Design review of the part built by this model. Coordinates are the model's own, in mm. Face numbers are marked on the shaded views. A direction names the side the tool comes from. Give positions to 0.01 mm unless a question says otherwise; leave off trailing zeros. Write each loop counter-clockwise with the first axis right and the second up, starting at its lowest first coordinate (ties: lowest second). Pieces come first, ordered by that corner, then holes. Notation, with made-up numbers: (42, 20) -> (80, 20) arc R17 ccw to (80, 50) -> close; hole circle Ø5 at (10.5, 36). An arc over 180 degrees is marked (long way). Answer as a JSON object with one key per item and string values.
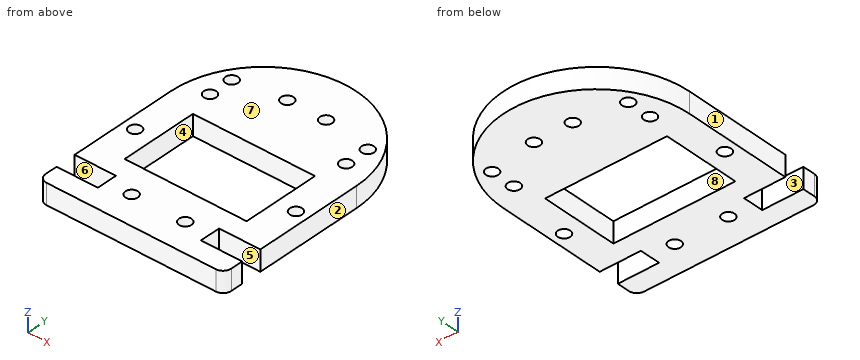
```python
from build123d import *

# Parameters (mm, degrees)
RESSALTO_EXTRUS_O2_DEPTH = 5
ESBO_O9_W                = 29.58
ESBO_O9_H                = 18.85
CORTE_EXTRUS_O1_DEPTH    = 5
ESBO_O10_R               = 1.5
CORTE_EXTRUS_O2_DEPTH    = 5
ESBO_O12_R               = 1.5
CORTE_EXTRUS_O3_DEPTH    = 10
ESBO_O13_R               = 1.5
CORTE_EXTRUS_O4_DEPTH    = 10
ESBO_O14_R               = 1.5
CORTE_EXTRUS_O5_DEPTH    = 76


with BuildPart() as part:
    # Esboço8 → Ressalto-extrusão2 (new body)
    with BuildSketch(Plane.XY):
        with BuildLine():
            Line((-24.266341706, -3.25), (-24.266341706, 13.25))
            ThreePointArc((-24.266341706, 13.25), (-1.766341706, 35.75), (20.733658294, 13.25))
            Line((20.733658294, 13.25), (20.733658294, -3.222268622))
            Line((20.733658294, -3.222268622), (20.733658294, -3.25))
            Line((20.733658294, -3.25), (20.733658294, -13.25))
            Line((20.733658294, -13.25), (10.733658294, -13.25))
            Line((10.733658294, -13.25), (10.733658294, -18.25))
            Line((10.733658294, -18.25), (20.733658294, -18.25))
            Line((20.733658294, -18.25), (20.733658294, -21.25))
            ThreePointArc((20.733658294, -21.25), (20.147871857, -22.664213562), (18.733658294, -23.25))
            Line((18.733658294, -23.25), (-22.266341706, -23.25))
            ThreePointArc((-22.266341706, -23.25), (-23.680555268, -22.664213562), (-24.266341706, -21.25))
            Line((-24.266341706, -21.25), (-24.266341706, -18.25))
            Line((-24.266341706, -18.25), (-14.266341706, -18.25))
            Line((-14.266341706, -18.25), (-14.266341706, -13.25))
            Line((-14.266341706, -13.25), (-24.266341706, -13.25))
            Line((-24.266341706, -13.25), (-24.266341706, -3.25))
        make_face()
    extrude(amount=RESSALTO_EXTRUS_O2_DEPTH)

    # Esboço9 → Corte-extrusão1 (cut)
    with BuildSketch(Plane(origin=(0, 0, 0), x_dir=(-1, 0, 0), z_dir=(0, 0, -1))):
        with Locations((1.766341706, 1.175)):
            Rectangle(ESBO_O9_W, ESBO_O9_H)
    extrude(amount=-CORTE_EXTRUS_O1_DEPTH, mode=Mode.SUBTRACT)

    # Esboço10 → Corte-extrusão2 (cut)
    with BuildSketch(Plane(origin=(0, 0, 0), x_dir=(-1, 0, 0), z_dir=(0, 0, -1))):
        with Locations((-17.733658294, 0)):
            Circle(ESBO_O10_R)
        with Locations((21.266341706, 0)):
            Circle(ESBO_O10_R)
    extrude(amount=-CORTE_EXTRUS_O2_DEPTH, mode=Mode.SUBTRACT)

    # Esboço12 → Corte-extrusão3 (cut)
    with BuildSketch(Plane.XY.offset(5)):
        with Locations((4.733658294, -15.75)):
            Circle(ESBO_O12_R)
        with Locations((-8.266341706, -15.75)):
            Circle(ESBO_O12_R)
    extrude(amount=-CORTE_EXTRUS_O3_DEPTH, mode=Mode.SUBTRACT)

    # Esboço13 → Corte-extrusão4 (cut)
    with BuildSketch(Plane.XY.offset(5)):
        with Locations((2.933658294, 25.15)):
            Circle(ESBO_O13_R)
        with Locations((-6.466341706, 25.15)):
            Circle(ESBO_O13_R)
    extrude(amount=-CORTE_EXTRUS_O4_DEPTH, mode=Mode.SUBTRACT)

    # Esboço14 → Corte-extrusão5 (cut)
    with BuildSketch(Plane.XY.offset(5)):
        with Locations((14.733658294, 17.25)):
            Circle(ESBO_O14_R)
        with Locations((14.733658294, 23.25)):
            Circle(ESBO_O14_R)
        with Locations((-18.266341706, 23.25)):
            Circle(ESBO_O14_R)
        with Locations((-18.266341706, 17.25)):
            Circle(ESBO_O14_R)
    extrude(amount=-CORTE_EXTRUS_O5_DEPTH, mode=Mode.SUBTRACT)


solid = part.part
```
(1) We need section B-B, the plane z = 2.25. Give the number of separate pieces and of enclosed holes in the cut face, then the cut area to 3 significant figures.
Here are the results:
{"separate pieces": "1", "enclosed holes": "11", "area": "1,710 mm²"}
(2) The part is to be moulded in two halves that separate along X. For the marked faces 1, 2, 3 and 4, say which applies: +X half, -X half, draft (parallel to the pull), parting line (faces both ways), or undercut.
Here are the results:
{"face 1": "-X half", "face 2": "+X half", "face 3": "draft", "face 4": "undercut"}
(3) We need section D-D, the plane x = -15. State the section outline as (y, z) points.
Here are the results:
{"outline": "(-23.25, 0) -> (-18.25, 0) -> (-18.25, 5) -> (-23.25, 5) -> close; (-13.25, 0) -> (-8.25, 0) -> (-8.25, 5) -> (-13.25, 5) -> close; (10.6, 0) -> (31.45, 0) -> (31.45, 5) -> (10.6, 5) -> close"}
(4) For the marked faces 5, 6, 7 and 8, list the 3-axis set-ups (+Z, -Z, +X, -X, +Y, -Y) from which the entire face can be reached by the end or side of a thin tool; tool diameter is ignored.
Here are the results:
{"face 5": "+Z, -Z, +X", "face 6": "+Z, -Z, -X", "face 7": "+Z, +X, -X, +Y, -Y", "face 8": "+Z, -Z"}
(5) We need section C-C, the plane y = 10. State the section outline as (x, z) points.
Here are the results:
{"outline": "(-24.27, 0) -> (-16.56, 0) -> (-16.56, 5) -> (-24.27, 5) -> close; (13.02, 0) -> (20.73, 0) -> (20.73, 5) -> (13.02, 5) -> close"}
(6) We need section A-A, the plane y = 0. State the section outline as (x, z) points.
Here are the results:
{"outline": "(-24.27, 0) -> (-22.77, 0) -> (-22.77, 5) -> (-24.27, 5) -> close; (-19.77, 0) -> (-16.56, 0) -> (-16.56, 5) -> (-19.77, 5) -> close; (13.02, 0) -> (16.23, 0) -> (16.23, 5) -> (13.02, 5) -> close; (19.23, 0) -> (20.73, 0) -> (20.73, 5) -> (19.23, 5) -> close"}
(7) For line 1 along Y through (x, z) = (18, 2.2); line 2 along Y through (x, z) = (-22, 0.9); line 3 along Y through (x, z) = (-7, 2.1), list the stretches that pass through material, from the lowest coordinate up.
Here are the results:
{"line 1": "y = -23.25 to -18.25, -13.25 to -1.48, 1.48 to 24", "line 2": "y = -23.25 to -18.25, -13.25 to -1.31, 1.31 to 23.09", "line 3": "y = -23.25 to -16.55, -14.95 to -8.25, 10.6 to 23.75, 26.55 to 35.13"}
(8) Clearance check with flat-ended pins moving along their axes: pin 1 (1.5 mm diameter, centred on y = -15.5, z = 1.5, fed in from +X); pin 2 (2.5 mm diameter, centred on x = 14.73, y = 23.25, fed in from +Z); pin 3 (2 mm diameter, centred on y = 15, z = 2.5, fed in from -X); pin 4 (1.5 mm diameter, centred on x = -3.5, z = 2, fed in from +Y). State where each tip first meets the part, or that it passes through.
Here are the results:
{"pin 1": "stops at x = 10.73", "pin 2": "passes through", "pin 3": "stops at x = -24.25", "pin 4": "stops at y = 35.73"}
